The model under review builds one solid part; all positions refer to its coordinate system, in mm. Coordinates: 2 decimals unless noted, no trailing zeros. Order: outer loops, then holes, each group sorted by start corner. A loop starts at its lowest first (then second) coordinate and runs counter-clockwise, first axis right, second up.
from build123d import *

# Parameters (mm, degrees)
F0_R     = 2.5
F1_DEPTH = 16.5
F2_R     = 2
F3_DEPTH = 16.501
F4_SIZE  = 0.1


with BuildPart() as f1:
    # F0 (on Top) → F1 (new body)
    with BuildSketch(Plane.XY):
        Circle(F0_R)
    extrude(amount=F1_DEPTH)

    # F2 (on face) → F3 (cut, through all)
    with BuildSketch(Plane.XY.offset(16.5)):
        Circle(F2_R)
    extrude(amount=-F3_DEPTH, mode=Mode.SUBTRACT)

    # F4
    f4_edges = [f1.edges().sort_by_distance(p)[0] for p in [
        (-2, 0, 0),
        (-2.5, 0, 0),
        (-2.5, 0, 16.5),
        (-2, 0, 16.5),
    ]]
    chamfer(f4_edges, length=F4_SIZE)


solid = f1.part
(1) Insertion check: pin 1 Ø1.5 at (x, z) = (1, 12.5) entering from +Y. The pin has a flat end and moves straight along its axis. Give the tip position at first contact, or say it passes through.
(2) Wall thickness on line 1 (Y direction, x = 0, z = 7.25); line 2 (X direction, y = 0.7, z = 1): over which ranges is each line inside the solid? List them lowest first.
(3) Consider section A-A (y = 0). Give the boundary of the cut face in (x, z), then the cut area to 3 significant figures.
(4) The part is to be moulded in two halves that separate along X. For faces 1 (the face through (0, -2, 8)), 2 (the face through (-0.54, -2.44, 8.14)), say which applies: +X half, -X half, draft (parallel to the pull), parting line (faces both ways), or undercut.
(5) Consider section C-C (z = 9.5). Give the boundary of the cut face in (x, y).
Findings:
1. pin 1: stops at y = 2.49
2. line 1: y = -2.5 to -2, 2 to 2.5
2. line 2: x = -2.4 to -1.87, 1.87 to 2.4
3. outline: (-2.5, 0.1) - (-2.4, 0) - (-2.1, 0) - (-2, 0.1) - (-2, 16.4) - (-2.1, 16.5) - (-2.4, 16.5) - (-2.5, 16.4) - close; (2, 0.1) - (2.1, 0) - (2.4, 0) - (2.5, 0.1) - (2.5, 16.4) - (2.4, 16.5) - (2.1, 16.5) - (2, 16.4) - close
3. area: 16.5 mm2
4. face 1: undercut
4. face 2: parting line
5. outline: circle Ø5 at (0, 0); hole circle Ø4 at (0, 0)
